Source: CAD feature listing. Evaluate the final solid. Frame: model axes, mm. A direction names the side the tool comes from. Give positions to 0.01 mm unless a question says otherwise; leave off trailing zeros. Loops run counter-clockwise (first coordinate to the right, second up) from the corner with the lowest first, then second, coordinate; pieces in that order, holes last. Notation, with made-up numbers: (11.25, 23.5) -> (59.25, 23.5) arc R28 ccw to (59.25, 45.5) -> close; hole circle Ø11 at (23.5, -27.75). An arc over 180 degrees is marked (long way). Put each result on its own line as item: value.
```python
from build123d import *

# Parameters (mm, degrees)
BOSS_EXTRUDE1_DEPTH              = 20
F_1_8_0_125_DIAMETER_HOLE1_D     = 3.175
F_1_8_0_125_DIAMETER_HOLE1_DEPTH = 9.69615506
FILLET1_R                        = 10


with BuildPart() as part:
    # Sketch1 → Boss-Extrude1 (new body)
    with BuildSketch(Plane.XY.offset(20)):
        with BuildLine():
            Line((-121.03432752, -152.461637247), (-121.18624999, -144.077694208))
            Line((-121.18624999, -144.077694208), (-121.18624999, -104.077694208))
            ThreePointArc((-121.18624999, -104.077694208), (-122.68624999, -102.577694208), (-124.18624999, -104.077694208))
            Line((-124.18624999, -104.077694208), (-124.18624999, -144.077694208))
            Line((-124.18624999, -144.077694208), (-130.88240505, -154.198119024))
            ThreePointArc((-130.88240505, -154.198119024), (-100.100592151, -207.513782914), (-42.249707279, -228.569783034))
            Line((-42.249707279, -228.569783034), (-32.249707279, -228.569783034))
            ThreePointArc((-32.249707279, -228.569783034), (-27.249707279, -223.569783034), (-32.249707279, -218.569783034))
            Line((-32.249707279, -218.569783034), (-42.249707279, -218.569783034))
            ThreePointArc((-42.249707279, -218.569783034), (-93.672716054, -199.853338483), (-121.03432752, -152.461637247))
        make_face()
    extrude(amount=-BOSS_EXTRUDE1_DEPTH)

    # 1/8 (0.125) Diameter Hole1
    with Locations(Plane(origin=(-121.18624999, 0, 0), x_dir=(0, 0, -1), z_dir=(1, 0, 0))):
        with Locations((-10, -120.077694208), (-10, -110.077694208)):
            Hole(F_1_8_0_125_DIAMETER_HOLE1_D / 2, depth=F_1_8_0_125_DIAMETER_HOLE1_DEPTH)

    # Fillet1
    fillet1_edges = [part.edges().sort_by_distance(p)[0] for p in [
        (-130.88240505, -154.198119024, 10),
        (-124.18624999, -144.077694208, 10),
        (-121.03432752, -152.461637247, 10),
    ]]
    fillet(fillet1_edges, radius=FILLET1_R)


solid = part.part
```
(1) First-contact query: P1, Ø1, axis at x = -51.5, z = 17.5, coming from the -Y side; P2, Ø8, axis at y = -160.5, z = 11, coming from the +X side; P3, Ø10, axis at x = -52.5, z = 12.5, coming from the -Y side. Flat tips, straight axial feed; report the tip coordinate or a pass-through.
Calculated:
P1: stops at y = -228.14
P2: stops at x = -117.93
P3: stops at y = -228.42
(2) Draft query along Z for faces 4 (the cylindrical face through (-27.25, -223.68, 10.14)), 5 (the cylindrical face through (-122.71, -121.63, 9.66)), 6 (the cylindrical face through (-122.71, -111.63, 9.66)), 7 (the flat face through (-90, -203, 20)). Return one class per face: released by +Z, released by -Z, zero draft, split by the parting line, or undercut.
Calculated:
face 4: zero draft
face 5: undercut
face 6: undercut
face 7: released by +Z
(3) Section D-D on x = -37. Return loops of the section in (y, z).
Calculated:
outline: (-228.57, 0) -> (-218.57, 0) -> (-218.57, 20) -> (-228.57, 20) -> close
(4) Line query: probe 1 along Y at (x, z) = (-123.4, 10); probe 2 along Y at (x, z) = (-122.95, 10); probe 3 along X at (y, z) = (-139, 19). Output: solid intervals per line, ascending. Write a range as from..to.
Calculated:
probe 1: y = -177.49..-121.67, -118.49..-111.67, -108.49..-102.76
probe 2: y = -178.41..-121.67, -118.49..-111.67, -108.49..-102.6
probe 3: x = -124.19..-121.19
(5) Section A-A on z = 10. Return loops of the section in (x, y), then the cut area to 3 significant figures.
Calculated:
outline: (-130.02, -158.49) arc R90 ccw to (-42.25, -228.57) -> (-32.25, -228.57) arc R5 ccw to (-32.25, -218.57) -> (-42.25, -218.57) arc R80 cw to (-120.88, -153.31) arc R10 cw to (-121.05, -151.65) -> (-121.19, -144.08) -> (-121.19, -121.67) -> (-124.19, -121.67) -> (-124.19, -141.07) arc R10 cw to (-125.85, -146.59) -> (-128.61, -150.76) arc R10 ccw to start; (-124.19, -118.49) -> (-121.19, -118.49) -> (-121.19, -111.67) -> (-124.19, -111.67) -> close; (-124.19, -108.49) -> (-121.19, -108.49) -> (-121.19, -104.08) arc R1.5 ccw to (-124.19, -104.08) -> close
area: 1,490 mm²
(6) Section B-B on z = 3. Return loops of the section in (x, y).
Calculated:
outline: (-130.02, -158.49) arc R90 ccw to (-42.25, -228.57) -> (-32.25, -228.57) arc R5 ccw to (-32.25, -218.57) -> (-42.25, -218.57) arc R80 cw to (-120.88, -153.31) arc R10 cw to (-121.05, -151.65) -> (-121.19, -144.08) -> (-121.19, -104.08) arc R1.5 ccw to (-124.19, -104.08) -> (-124.19, -141.07) arc R10 cw to (-125.85, -146.59) -> (-128.61, -150.76) arc R10 ccw to start
(7) Reachability of faces 1 (the flat face through (-37, -218.57, 10)), 2 (the cylindrical face through (-122.65, -102.58, 10.14)), 3 (the flat face through (-124.186, -122, 10)) from +Z, -Z, +X, -X, +Y, -Y: full face, straight path, thin tool, end or side. Return the list, or none.
Calculated:
face 1: +Z, -Z, +X, +Y
face 2: +Z, -Z, +Y
face 3: +Z, -Z, -X, +Y
(8) Section C-C on y = -130. Return loops of the section in (x, z), then the cut area to 3 significant figures.
Calculated:
outline: (-124.19, 0) -> (-121.19, 0) -> (-121.19, 20) -> (-124.19, 20) -> close
area: 60.0 mm²
